Check sheet for the modelled part. Datum: model origin and axes. Units: mm. Face numbers are marked on the shaded views. A direction names the side the tool comes from. Give positions to 0.01 mm unless a question says otherwise; leave off trailing zeros. Order: outer loops, then holes, each group sorted by start corner. A loop starts at its lowest first (then second) coordinate and runs counter-clockwise, first axis right, second up.
from build123d import *

# Parameters (mm, degrees)
F1_DEPTH = 250
F2_R     = 6
F3_DEPTH = 80.001


with BuildPart() as f1:
    # F0 (on Top) → F1 (new body, symmetric)
    with BuildSketch(Plane.XY):
        with BuildLine():
            Line((0, 110), (0, 0))
            Line((0, 0), (80, 0))
            Line((80, 0), (80, 2.233367))
            ThreePointArc((80, 2.233367), (78.362298, 6.547073), (74.274444, 8.687067))
            Line((74.274444, 8.687067), (20.010685, 15.198718))
            ThreePointArc((20.010685, 15.198718), (12.149427, 19.31409), (9, 27.609678))
            Line((9, 27.609678), (9, 110))
            Line((9, 110), (9, 192.390322))
            ThreePointArc((9, 192.390322), (12.149427, 200.68591), (20.010685, 204.801282))
            Line((20.010685, 204.801282), (74.274444, 211.312933))
            ThreePointArc((74.274444, 211.312933), (78.362298, 213.452927), (80, 217.766633))
            Line((80, 217.766633), (80, 220))
            Line((80, 220), (0, 220))
            Line((0, 220), (0, 110))
        make_face()
    extrude(amount=F1_DEPTH, both=True)

    # F2 (on face) → F3 (cut, through all)
    with BuildSketch(Plane(origin=(0, 0, 0), x_dir=(0, -1, 0), z_dir=(-1, 0, 0))):
        with Locations((-70, 210)):
            Circle(F2_R)
        with Locations((-150, 210)):
            Circle(F2_R)
        with Locations((-70, 130)):
            Circle(F2_R)
        with Locations((-150, 130)):
            Circle(F2_R)
    extrude(amount=-F3_DEPTH, mode=Mode.SUBTRACT)


solid = f1.part
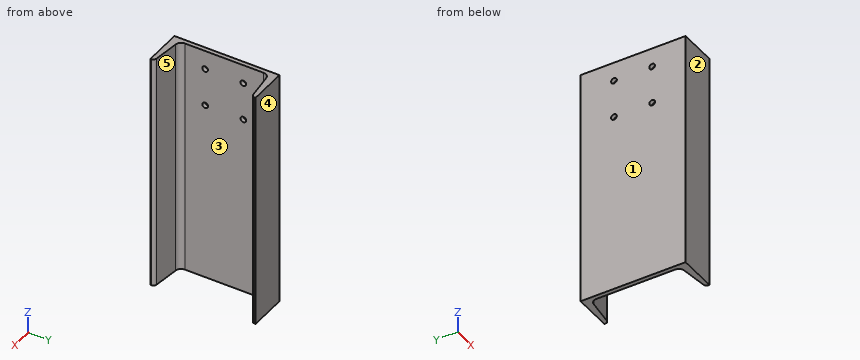
1) Draft check along Y on the marked faces 1, 2 and 3. Enter one of: +Y half, -Y half, draft (parallel to the pull), parting line (faces both ways), or undercut.
Recorded:
face 1: draft
face 2: -Y half
face 3: undercut
2) Section check B-B, the plane y = 150. Record the cut outline in (x, z).
Recorded:
outline: (0, -250) - (9, -250) - (9, 124) - (0, 124) - close; (0, 136) - (9, 136) - (9, 204) - (0, 204) - close; (0, 216) - (9, 216) - (9, 250) - (0, 250) - close
3) Section check C-C, the plane z = 210. Record the cut outline in (x, y).
Recorded:
outline: (0, 0) - (80, 0) - (80, 2.23) arc R6.5 ccw to (74.27, 8.69) - (20.01, 15.2) arc R12.5 cw to (9, 27.61) - (9, 64) - (0, 64) - close; (0, 76) - (9, 76) - (9, 144) - (0, 144) - close; (0, 156) - (9, 156) - (9, 192.39) arc R12.5 cw to (20.01, 204.8) - (74.27, 211.31) arc R6.5 ccw to (80, 217.77) - (80, 220) - (0, 220) - close
4) Set-up check for the marked faces 4 and 5: record each of +Z, -Z, +X, -X, +Y, -Y from which the full face is reachable in a straight line by a thin tool's end or side.
Recorded:
face 4: +Z, -Z, +X, -X, +Y
face 5: +Z, -Z, +X
5) Depth check by flat-ended pin: pin 1 Ø10 at (x, z) = (22.5, 105) entering from -Y; pin 2 Ø15.5 at (y, z) = (150, 130) entering from +X. Enter the tip coordinate at first touch or a pass-through.
Recorded:
pin 1: stops at y = 0
pin 2: stops at x = 9
6) Material ranges on L1, parallel to Z at x = 6, y = 150; L2, parallel to Y at x = 20, z = 158.5; L3, parallel to Y at x = 48, z = -101, recorded low to high.
Recorded:
L1: z = -250 to 124, 136 to 204, 216 to 250
L2: y = 0 to 15.2, 204.8 to 220
L3: y = 0 to 11.84, 208.16 to 220
7) Section check A-A, the plane x = 31.5. Record the cut outline in (y, z).
Recorded:
outline: (0, -250) - (13.82, -250) - (13.82, 250) - (0, 250) - close; (206.18, -250) - (220, -250) - (220, 250) - (206.18, 250) - close
8) Section check D-D, the plane z = 30. Record the cut outline in (x, y).
Recorded:
outline: (0, 0) - (80, 0) - (80, 2.23) arc R6.5 ccw to (74.27, 8.69) - (20.01, 15.2) arc R12.5 cw to (9, 27.61) - (9, 192.39) arc R12.5 cw to (20.01, 204.8) - (74.27, 211.31) arc R6.5 ccw to (80, 217.77) - (80, 220) - (0, 220) - close
